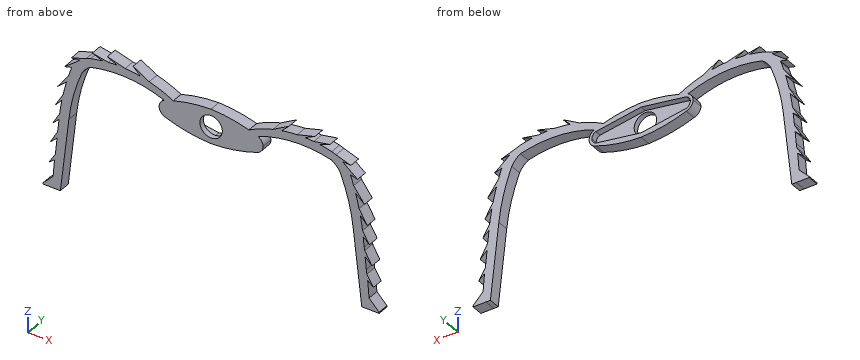
```python
from build123d import *

# Parameters (mm, degrees)
PAD034_DEPTH       = 4
PAD032_DEPTH       = 4
POCKET003027_DEPTH = 2.2
PAD033_DEPTH       = 4
SKETCH054_R        = 3.9
POCKET003028_DEPTH = 10


with BuildPart() as central_leg_insect_add:
    # Sketch055 → Pad034 (new body)
    with BuildSketch(Plane.XZ.offset(-43.7)):
        Polygon((-58.503296, -18.004301), (-53.997036, -18.004301), (-48.744877, 15.965196), (-44.5658, 27.943165), (-41.53833, 30.02603), (-31.626242, 31.40176), (-21.017805, 29.65671), (-18.990362, 30.401161), (-27.13097, 35.111233), (-22.936073, 30.916338), (-29.003351, 32.984856), (-36.116627, 34.99157), (-32.000511, 32.969288), (-34.972557, 32.969288), (-41.352551, 34.221657), (-37, 32.591213), (-43, 31.631081), (-48.636986, 29.73181), (-44, 30.22826), (-46, 29.721722), (-51, 25.793291), (-47.464714, 26.759798), (-49.314915, 23.492535), (-53.390827, 18), (-50, 21), (-51, 16.646269), (-54.355499, 11), (-51.685394, 14), (-52.498241, 9), (-55.106018, 4.606695), (-52.495518, 7), (-53.502594, 2), (-56, -2.398534), (-53.492668, 0), (-54.22747, -6), (-56.500393, -9.69598), (-54.497387, -8), (-55, -14), (-58.503296, -17.601286), align=None)
    extrude(amount=-PAD034_DEPTH)


with BuildPart() as quarter_central_leg_servo_support:
    # Sketch050 → Pad032 (new body)
    with BuildSketch(Plane(origin=(0, 47.7, 24.6), x_dir=(-1, 0, 0), z_dir=(0, 1, 0))):
        with BuildLine():
            ThreePointArc((15.732627, 3), (7.987175, 5.135172), (0, 6.004658))
            Line((0, 6.004658), (0, 4.275313))
            Line((0, 4.275313), (0, 0))
            Line((16.774147, 0), (0, 0))
            Line((18.088162, 0), (16.774147, 0))
            ThreePointArc((18.088162, 0), (17.428911, 1.907128), (15.732627, 3))
        make_face()
    extrude(amount=-PAD032_DEPTH)

    # Sketch051 → Pocket003027 (cut)
    with BuildSketch(Plane(origin=(0, 47.7, 24.6), x_dir=(-1, 0, 0), z_dir=(0, 1, 0))):
        with BuildLine():
            Line((0, 4.49111), (15.744728, 2.000001))
            ThreePointArc((17.134156, 0), (16.75271, 1.217632), (15.744728, 2.000001))
            Line((17.134156, 0), (0, 0))
            Line((0, 0), (0, 4.49111))
        make_face()
    extrude(amount=-POCKET003027_DEPTH, mode=Mode.SUBTRACT)


with BuildPart() as half_leg_insect:
    # Part__Mirroring001: instance of quarter_central_leg_servo_support
    add(quarter_central_leg_servo_support.part.mirror(Plane(origin=(0, 0, 24.6), x_dir=(0, 1, 0), z_dir=(0, 0, 1))))

    # Fusion007017: union quarter_central_leg_servo_support
    add(quarter_central_leg_servo_support.part)

    # Sketch052 → Pad033 (new body)
    with BuildSketch(Plane(origin=(0, 47.7, 0), x_dir=(-1, 0, 0), z_dir=(0, 1, 0))):
        with BuildLine():
            Line((52.452988, -18.000002), (58.497849, -18.000002))
            Line((58.497849, -18.000002), (58.497849, -17.584217))
            ThreePointArc((54.988709, -14), (56.535613, -15.995425), (58.497849, -17.584217))
            Line((54.988709, -14), (52.759255, 8.35829))
            ThreePointArc((52.759255, 8.35829), (51.202034, 17.133916), (48.77817, 25.710712))
            ThreePointArc((48.77817, 25.710712), (46.1643, 29.690829), (42.000002, 32))
            ThreePointArc((42.000002, 32), (27.145674, 33.002324), (13.00001, 28.359486))
            Line((16, 27.29138), (13.00001, 28.359486))
            ThreePointArc((41.999998, 28.999997), (28.860359, 30.270585), (16, 27.29138))
            ThreePointArc((44.999996, 25.769916), (43.714535, 27.584213), (41.999998, 28.999997))
            ThreePointArc((49.501895, 8.000017), (47.87481, 17.043019), (44.999996, 25.769916))
            Line((52.452988, -18.000002), (49.501895, 8.000017))
        make_face()
    extrude(amount=-PAD033_DEPTH)

    # Fusion007018: union central_leg_insect_add
    add(central_leg_insect_add.part)


with BuildPart() as obj1:
    # Part__Mirroring002: instance of half_leg_insect
    add(half_leg_insect.part.mirror(Plane(origin=(0, 0, 0), x_dir=(0, -1, 0), z_dir=(1, 0, 0))))

    # Fusion007019: union half_leg_insect
    add(half_leg_insect.part)

    # Sketch054 → Pocket003028 (cut)
    with BuildSketch(Plane(origin=(0, 45.5, 0), x_dir=(-1, 0, 0), z_dir=(0, 1, 0))):
        with Locations((0, 24.473736)):
            Circle(SKETCH054_R)
    extrude(amount=-POCKET003028_DEPTH, mode=Mode.SUBTRACT)


solid = obj1.part
```
Could you check a few things on this model? Use its own coordinates, in mm. Round coordinates to 2 decimals unless told otherwise and drop trailing zeros. Loops run counter-clockwise (first coordinate to the right, second up) from the corner with the lowest first, then second, coordinate; pieces in that order, holes last. Notation, with made-up numbers: M 28,82 L 46,82 A23 ccw 46,98 Z; hole C -22,89 d10. An arc over 180 degrees is marked long. Answer as CSV lines item,"result".
1) If I drill on probe 1 along Z at (x, y) = (0, 44.65); probe 2 along Z at (x, y) = (14.5, 46.1); probe 3 along X at (y, z) = (46.5, 10), over which ranges is the centre line in solid material (lowest first)?
From the geometry:
probe 1,"18.6 to 20.57, 28.37 to 30.6"
probe 2,"21.17 to 22.4, 26.8 to 29.15"
probe 3,"-52.54 to -49.25, 49.25 to 52.54"
2) Imagine slicing it at A-A on z = -11. List the corners of the cut face in (x, y) for me, and give its area (3 significant figures).
From the geometry:
outline,"M -54.75,43.7 L -51.66,43.7 L -51.66,47.7 L -54.75,47.7 Z; M 51.66,43.7 L 54.75,43.7 L 54.75,47.7 L 51.66,47.7 Z"
area,"24.7 mm^2"
3) Imagine slicing it at B-B on x = 23. List the corners of the cut face in (y, z) for me.
From the geometry:
outline,"M 43.7,29.46 L 47.7,29.46 L 47.7,32.72 L 43.7,32.72 Z"
4) For pin 1 Ø2.5 at (x, z) = (-4.5, 27) entering from +Y; pin 2 Ø2 at (y, z) = (47, 17.5) entering from -X; pin 3 Ø1.2 at (x, y) = (-53, 45) entering from -Z, each with a flat end and sliding along its axis, tell me the tip position at first contact or that it passes through.
From the geometry:
pin 1,"y = 45.5"
pin 2,"x = -53.39"
pin 3,"z = -18"
